Check sheet for the drawn part. Datum: minimum x, y, z corner. Units: mm. A direction names the side the tool comes from. Round coordinates to 2 decimals unless told otherwise and drop trailing zeros. Write each loop counter-clockwise with the first axis right and the second up, starting at its lowest first coordinate (ties: lowest second). Pieces come first, ordered by that corner, then holes. Notation, with made-up numbers: (88.5, -8.75) -> (100.5, -8.75) arc R6 cw to (100.5, -4.75) -> close; hole circle Ø5 at (80, 89). An arc over 180 degrees is marked (long way). One line per item, written item: value.
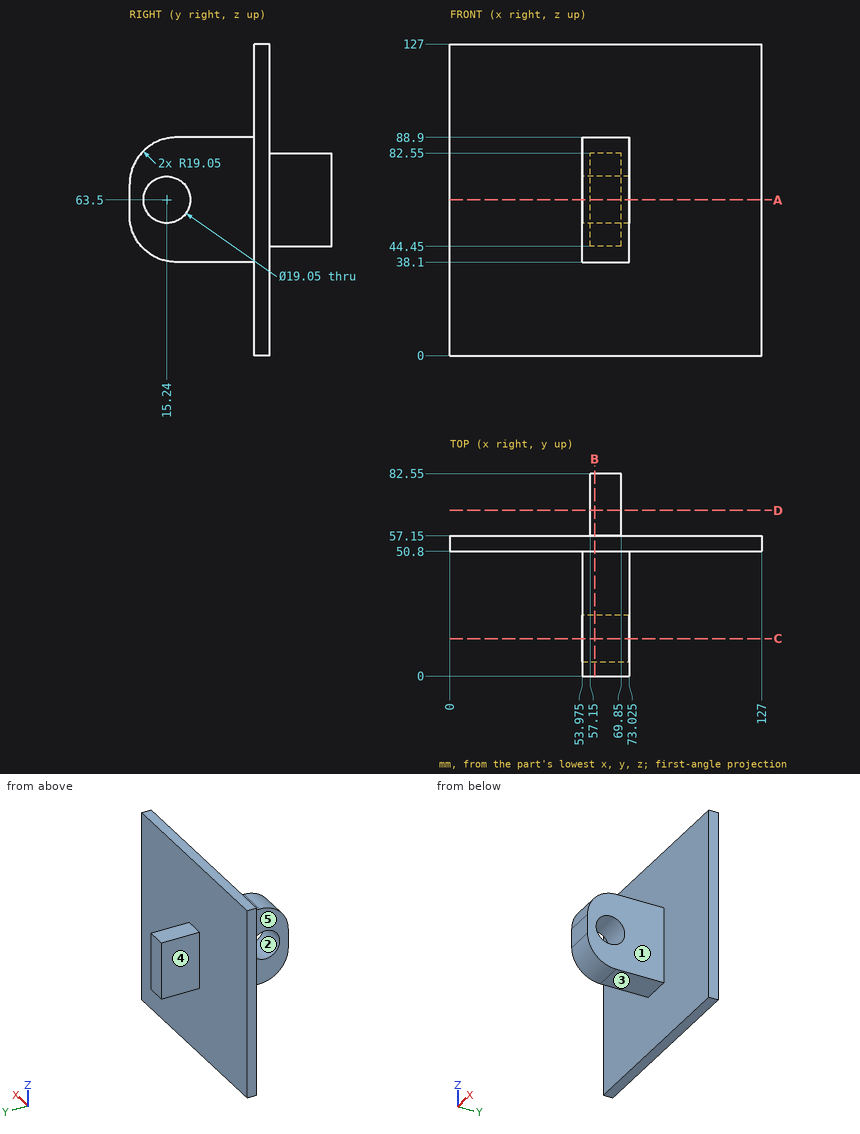
Item 1: Sectioned sample at A-A on z = 63.5. Enter the section's corners in (x, y) (3 decimals), and give its area (3 significant figures).
Answer:
outline: (0, 50.8) -> (53.975, 50.8) -> (53.975, 24.765) -> (73.025, 24.765) -> (73.025, 50.8) -> (127, 50.8) -> (127, 57.15) -> (69.85, 57.15) -> (69.85, 82.55) -> (57.15, 82.55) -> (57.15, 57.15) -> (0, 57.15) -> close; (53.975, 0) -> (73.025, 0) -> (73.025, 5.715) -> (53.975, 5.715) -> close
area: 1,730 mm^2
Item 2: Sectioned sample at D-D on y = 67.5. Enter the section's corners in (x, z).
Answer:
outline: (57.15, 44.45) -> (69.85, 44.45) -> (69.85, 82.55) -> (57.15, 82.55) -> close
Item 3: Sectioned sample at B-B on x = 59. Enter the section's corners in (y, z) (3 decimals).
Answer:
outline: (0, 57.15) arc R19.05 ccw to (19.05, 38.1) -> (50.8, 38.1) -> (50.8, 0) -> (57.15, 0) -> (57.15, 44.45) -> (82.55, 44.45) -> (82.55, 82.55) -> (57.15, 82.55) -> (57.15, 127) -> (50.8, 127) -> (50.8, 88.9) -> (19.05, 88.9) arc R19.05 ccw to (0, 69.85) -> close; hole circle Ø19.05 at (15.24, 63.5)
Item 4: Sectioned sample at C-C on y = 15.24. Enter the section's corners in (x, z) (3 decimals).
Answer:
outline: (53.975, 38.485) -> (73.025, 38.485) -> (73.025, 53.975) -> (53.975, 53.975) -> close; (53.975, 73.025) -> (73.025, 73.025) -> (73.025, 88.515) -> (53.975, 88.515) -> close
Item 5: Thickness scan on line 1 (Y direction, x = 69, z = 63); line 2 (Y direction, x = 116, z = 111.5); line 3 (X direction, y = 46, z = 46) (3 decimals). Record the ranges inside material, lowest first.
Answer:
line 1: y = 0 to 5.73, 24.75 to 82.55
line 2: y = 50.8 to 57.15
line 3: x = 53.975 to 73.025
Item 6: Depth check by flat-ended pin: P1, Ø1.5, axis at x = 65, y = 14, coming from the +Z side; P2, Ø15, axis at x = 62, y = 28, coming from the +Z side; P3, Ø2, axis at y = 45.5, z = 64, coming from the +X side (3 decimals); P4, Ø11.5, axis at y = 15.24, z = 63.5, coming from the +X side. Enter the tip coordinate at first touch or a pass-through.
Answer:
P1: stops at z = 88.41
P2: stops at z = 88.9
P3: stops at x = 73.025
P4: passes through
Item 7: Tool access check on the marked faces 1, 2, 3, 4 and 5. Record the directions out of +Z, -Z, +X, -X, +Y, -Y that give a thin tool (end or side, any length) a straight path to the whole face; none if there is none.
Answer:
face 1: +Z, -Z, +X, -Y
face 2: +X, -X
face 3: -Z, +X, -X, -Y
face 4: +Z, -Z, -X, +Y
face 5: +Z, -Z, -X, -Y
